For this review, use the dimensioned drawing (mm, ordinates from the lowest corner) and the shaded views. A direction names the side the tool comes from. Coordinates: 2 decimals unless noted, no trailing zeros. Loops run counter-clockwise (first coordinate to the right, second up) from the corner with the lowest first, then second, coordinate; pieces in that order, holes last. Notation, with made-up numbers: (5, -22) - (46, -22) arc R35 ccw to (46, 13) - close; hole circle Ø5 at (84.25, 9). An arc over 180 degrees is marked (long way). One line per item, written item: value. Start each with the question number.
1. We need section C-C, the plane z = 33. Give the boundary of the cut face in (x, y).
2. To check wall thickness, follow line 1 (X direction, y = 11.5, z = 8) (1 decimal); line 2 (Y direction, x = 11, z = 55.5); line 3 (Z direction, x = 53.5, y = 9). State the ranges of each line that lie inside material, in increasing order.
3. For the marked faces 1, 2 and 3, list the 3-axis set-ups (+Z, -Z, +X, -X, +Y, -Y) from which the entire face can be reached by the end or side of a thin tool; tool diameter is ignored.
4. We need section A-A, the plane y = 59.5. Give the boundary of the cut face in (x, z) (1 decimal).
5. We need section D-D, the plane x = 50.5. Give the boundary of the cut face in (y, z) (1 decimal), then the cut area to 3 significant figures.
6. Insertion check: P1, Ø6, axis at x = 76, y = 20.5, coming from the +Z side; P2, Ø5, axis at x = 78, z = 72, coming from the -Y side; P3, Ø10.5, axis at x = 58, y = 22.5, coming from the +Z side; P4, Ø8, axis at x = 53, y = 55, coming from the -Z side. Each pin has a flat end and moves straight along its axis. Give the tip position at first contact, or say it passes through.
7. We need section B-B, the plane y = 27. Give the boundary of the cut face in (x, z) (1 decimal).
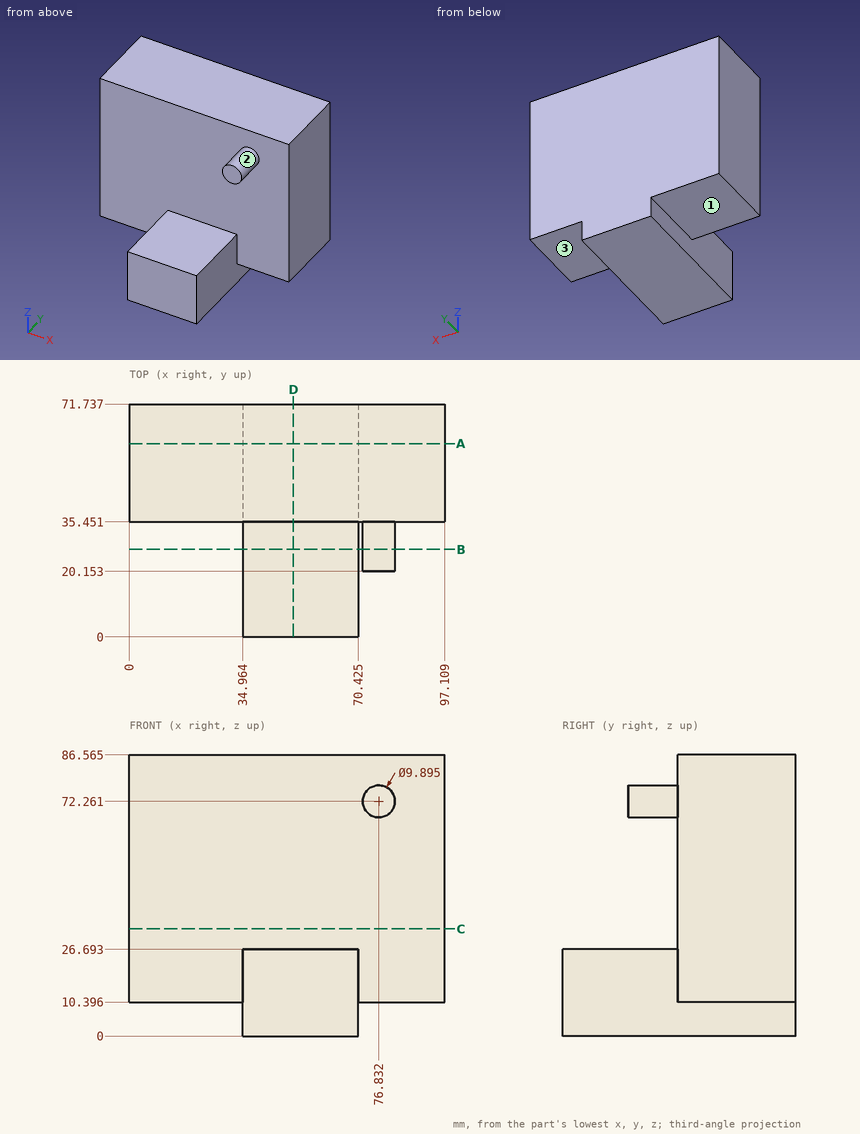
Findings below:
1. outline: (0, 35.45) - (97.11, 35.45) - (97.11, 71.74) - (0, 71.74) - close
2. line 1: 35 to 70.4
2. line 2: 35.45 to 71.74
2. line 3: 0 to 26.69
3. face 1: -Z, -X, +Y, -Y
3. face 2: -Y
3. face 3: -Z, +X, +Y, -Y
4. outline: (0, 10.4) - (35, 10.4) - (35, 0) - (70.4, 0) - (70.4, 10.4) - (97.1, 10.4) - (97.1, 86.6) - (0, 86.6) - close
5. outline: (0, 0) - (71.7, 0) - (71.7, 86.6) - (35.5, 86.6) - (35.5, 26.7) - (0, 26.7) - close
5. area: 4,090 mm2
6. P1: z = 77.21
6. P2: y = 20.15
6. P3: z = 26.69
6. P4: z = 0
7. outline: (35, 0) - (70.4, 0) - (70.4, 26.7) - (35, 26.7) - close; circle Ø9.9 at (76.8, 72.3)
